```python
from build123d import *

# Parameters (mm, degrees)
F0_R     = 5
F1_DEPTH = 5
F2_R     = 1


with BuildPart() as f1:
    # F0 (on Top) → F1 (new body)
    with BuildSketch(Plane.XY):
        with BuildLine():
            Line((28.5, -10), (36.5, -10))
            Line((36.5, -10), (36.5, 0))
            ThreePointArc((36.5, 0), (40, 3.5), (43.5, 0))
            Line((43.5, 0), (43.5, -9.3674969976))
            ThreePointArc((43.5, -9.3674969976), (48.2158383626, -5.7008771255), (50, 0))
            ThreePointArc((50, 0), (47.0710678119, 7.0710678119), (40, 10))
            Line((40, 10), (-40, 10))
            ThreePointArc((-40, 10), (-47.0710678119, 7.0710678119), (-50, 0))
            ThreePointArc((-50, 0), (-47.0710678119, -7.0710678119), (-40, -10))
            Line((-40, -10), (-23.5, -10))
            Line((-23.5, -10), (-23.5, 0))
            ThreePointArc((-23.5, 0), (-20, 3.5), (-16.5, 0))
            Line((-16.5, 0), (-16.5, -10))
            Line((-16.5, -10), (-8.5, -10))
            Line((-8.5, -10), (-8.5, 0))
            ThreePointArc((-8.5, 0), (-5, 3.5), (-1.5, 0))
            Line((-1.5, 0), (-1.5, -10))
            Line((-1.5, -10), (6.5, -10))
            Line((6.5, -10), (6.5, 0))
            ThreePointArc((6.5, 0), (10, 3.5), (13.5, 0))
            Line((13.5, 0), (13.5, -10))
            Line((13.5, -10), (21.5, -10))
            Line((21.5, -10), (21.5, 0))
            ThreePointArc((21.5, 0), (25, 3.5), (28.5, 0))
            Line((28.5, 0), (28.5, -10))
        make_face()
        with Locations((-40, 0)):
            Circle(F0_R, mode=Mode.SUBTRACT)
    extrude(amount=F1_DEPTH)

    # F2
    f2_edges = [f1.edges().sort_by_distance(p)[0] for p in [
        (-31.75, -10, 5),
        (-50, 0, 5),
        (-12.5, -10, 5),
        (2.5, -10, 5),
        (17.5, -10, 5),
        (32.5, -10, 5),
        (49.840604, 1.778346, 5),
        (0, 10, 5),
        (-45, 0, 5),
        (-23.5, -5, 5),
        (-20, 3.5, 5),
        (-16.5, -5, 5),
        (-8.5, -5, 5),
        (6.5, -5, 5),
        (21.5, -5, 5),
        (40, 3.5, 5),
    ]]
    fillet(f2_edges, radius=F2_R)


solid = f1.part
```
Check sheet for the modelled part. Datum: model origin and axes. Units: mm. A direction names the side the tool comes from. Round coordinates to 2 decimals unless told otherwise and drop trailing zeros. Order: outer loops, then holes, each group sorted by start corner. A loop starts at its lowest first (then second) coordinate and runs counter-clockwise, first axis right, second up. Notation, with made-up numbers: (32, 80.5) -> (42, 80.5) arc R12 ccw to (42, 91.5) -> close; hole circle Ø8 at (30.25, 6.5). An arc over 180 degrees is marked (long way). One line per item, written item: value. Start each with the question number.
Q1. Cross-section at C-C (y = 1.5). Give the number of separate pieces and of enclosed holes in the cut face, and give its area (3 significant figures).
Q2. Cross-section at B-B (x = -20). Record the boundary of the cut face in (y, z).
Q3. Set-up check for faces 1 (the face through (-32, -10, 2)), 2 (the face through (36.5, -5, 2)): record each of +Z, -Z, +X, -X, +Y, -Y from which the full face is reachable in a straight line by a thin tool's end or side.
Q4. Mould release check, pull along X, two halves, no side actions. Record for faces 3 (the face through (17, -10, 2)), 4 (the face through (13.5, -5, 2)): pulls with the +X half, pulls with the -X half, needs draft (parallel to the pull), parting line crosses it, or undercut.
Q5. Thickness scan on line 1 (Y direction, x = -40, z = 2.4); line 2 (X direction, y = -7.75, z = 3.6); line 3 (X direction, y = -6.25, z = 2.8). Record the ranges inside material, lowest first.
Q6. Gauge pin test, flat ends, axial feed: pin 1 Ø3 at (y, z) = (-4.5, 1.5) entering from +X; pin 2 Ø1.2 at (y, z) = (-4, 1.5) entering from +X; pin 3 Ø3 at (y, z) = (-2.5, 4) entering from -X. Record the tip position at first contact, or that the pin passes through.
Q7. Cross-section at A-A (z = 3). Record the boundary of the cut face in (x, y), and give its area (3 significant figures).
Completed:
1. separate pieces: 7
1. enclosed holes: 0
1. area: 290 mm²
2. outline: (3.5, 0) -> (10, 0) -> (10, 4) arc R1 ccw to (9, 5) -> (4.5, 5) arc R1 ccw to (3.5, 4) -> close
3. face 1: +Z, -Z, +X, -X, -Y
3. face 2: +Z, -Z, -Y
4. face 3: needs draft
4. face 4: undercut
5. line 1: y = -10 to -5, 5 to 10
5. line 2: x = -46.32 to -23.5, -16.5 to -8.5, -1.5 to 6.5, 13.5 to 21.5, 28.5 to 36.5, 43.5 to 46.32
5. line 3: x = -47.81 to -23.5, -16.5 to -8.5, -1.5 to 6.5, 13.5 to 21.5, 28.5 to 36.5, 43.5 to 47.81
6. pin 1: stops at x = 49.54
6. pin 2: stops at x = 49.4
6. pin 3: stops at x = -49.95
7. outline: (-40, -10) -> (-23.5, -10) -> (-23.5, 0) arc R3.5 cw to (-16.5, 0) -> (-16.5, -10) -> (-8.5, -10) -> (-8.5, 0) arc R3.5 cw to (-1.5, 0) -> (-1.5, -10) -> (6.5, -10) -> (6.5, 0) arc R3.5 cw to (13.5, 0) -> (13.5, -10) -> (21.5, -10) -> (21.5, 0) arc R3.5 cw to (28.5, 0) -> (28.5, -10) -> (36.5, -10) -> (36.5, 0) arc R3.5 cw to (43.5, 0) -> (43.5, -9.37) arc R10 ccw to (40, 10) -> (-40, 10) arc R10 ccw to start; hole circle Ø10 at (-40, 0)
7. area: 1,390 mm²
